Job drawing, mm, ordinate dimensions from the low corner. One solid piece. A direction names the side the tool comes from. Give positions to 0.01 mm unless a question says otherwise; leave off trailing zeros. Order: outer loops, then holes, each group sorted by start corner. A loop starts at its lowest first (then second) coordinate and runs counter-clockwise, first axis right, second up. Notation, with made-up numbers: M 61.25,-8.5 L 100.25,-8.5 A21 ccw 100.25,27.5 Z; hole C 79.25,-34.75 d9. An arc over 180 degrees is marked long. Use CSV: the item, a comma, the result in double quotes. Start each with the question number.
Item 1: Two-plate mould, pull along Z, no slides. Class the marked faces 1, 2 and 3: pulls with the +Z half, pulls with the -Z half, needs draft (parallel to the pull), parting line crosses it, or undercut.
Item 2: Which spindle directions (+Z, -Z, +X, -X, +Y, -Y) get a long thin tool onto all of the face, cutting with end or side? Do the marked faces 4, 5 and 6. Say none if no direction does.
Item 3: Band-saw the part on B-B on y = 60. Write the cut outline in (x, z), plus the area to 4 significant figures.
Item 4: Band-saw the part on A-A on z = 60. Write the cut outline in (x, y).
Item 5: Band-saw the part on C-C on x = 7. Give the number of separate pieces and of enclosed holes in the cut face, plus the area to 3 significant figures.
Item 6: Band-saw the part on D-D on x = 25.75. Write the cut outline in (y, z).
Item 7: Pin check, flat tips, straight feed: P1, Ø14.5, axis at y = 44.55, z = 12.45, coming from the +X side; P2, Ø6, axis at x = 12.5, y = 15, coming from the -Z side; P3, Ø7, axis at y = 44.55, z = 107.55, coming from the +X side; P4, Ø10, axis at x = 9.5, z = 95.5, coming from the -Y side. Stop position of each tip, or through.
Item 8: Wall check: line 1 along Y through (x, z) = (3, 94.5) (1 decimal); line 2 along Y through (x, z) = (20.25, 57.5) (1 decimal); line 3 along Z through (x, y) = (3, 8) (1 decimal). Give the ranges that are in metal, low to high.
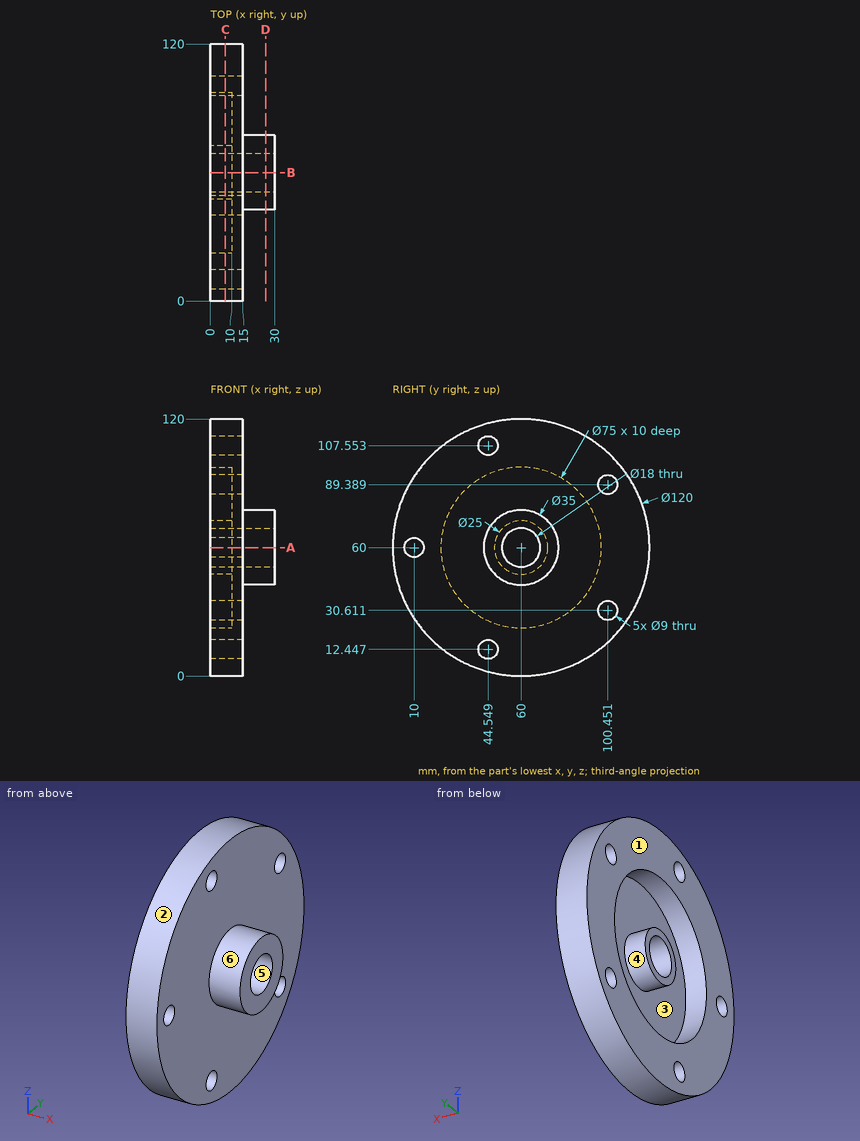
Model answer:
1,face 1,"needs draft"
1,face 2,"parting line crosses it"
1,face 3,"undercut"
2,face 4,"-X"
2,face 5,"+X, -X"
2,face 6,"+X"
3,outline,"M 0,0 L 15,0 L 15,42.5 L 30,42.5 L 30,51 L 0,51 L 0,47.5 L 10,47.5 L 10,22.5 L 0,22.5 Z; M 0,69 L 30,69 L 30,77.5 L 15,77.5 L 15,120 L 0,120 L 0,97.5 L 10,97.5 L 10,72.5 L 0,72.5 Z"
3,area,"1,285 mm^2"
4,outline,"M 0,0 L 15,0 L 15,5.5 L 0,5.5 Z; M 0,14.5 L 15,14.5 L 15,42.5 L 30,42.5 L 30,51 L 0,51 L 0,47.5 L 10,47.5 L 10,22.5 L 0,22.5 Z; M 0,69 L 30,69 L 30,77.5 L 15,77.5 L 15,120 L 0,120 L 0,97.5 L 10,97.5 L 10,72.5 L 0,72.5 Z"
5,separate pieces,"2"
5,enclosed holes,"7"
5,area,"6,810 mm^2"
6,outline,"C 60,60 d35; hole C 60,60 d18"
7,P1,"stops at x = 15"
7,P2,"stops at z = 17.15"
7,P3,"passes through"
7,P4,"stops at y = 8.33"
8,line 1,"y = 10.9 to 45.3, 74.7 to 109.1"
8,line 2,"y = 42.7 to 51.4, 68.6 to 77.3"
8,line 3,"z = 30.1 to 56, 64 to 89.9"
